```python
from build123d import *

# Parameters (mm, degrees)
F0_W     = 80
F0_H     = 25
F0_R     = 2.75
F1_DEPTH = 10
F2_R     = 4
F3_R     = 2


with BuildPart() as f1:
    # F0 (on Top) → F1 (new body)
    with BuildSketch(Plane.XY):
        Rectangle(F0_W, F0_H)
        with Locations((32.5, 0)):
            Circle(F0_R, mode=Mode.SUBTRACT)
    extrude(amount=F1_DEPTH)

    # F2
    f2_edges = [f1.edges().sort_by_distance(p)[0] for p in [
        (40, -12.5, 5),
        (-40, -12.5, 5),
        (40, 12.5, 5),
        (-40, 12.5, 5),
    ]]
    fillet(f2_edges, radius=F2_R)

    # F3
    f3_edges = [f1.edges().sort_by_distance(p)[0] for p in [
        (0, -12.5, 10),
    ]]
    fillet(f3_edges, radius=F3_R)


solid = f1.part
```
Could you check a few things on this model? Use its own coordinates, in mm. Round coordinates to 2 decimals unless told otherwise and drop trailing zeros. Loops run counter-clockwise (first coordinate to the right, second up) from the corner with the lowest first, then second, coordinate; pieces in that order, holes last.
Q1. I want a section at A-A (y = 0). Write out the boundary of the cut face in (x, z).
Q2. I want a section at C-C (z = 3.75). Write out the boundary of the cut face in (x, y), and give its area (3 significant figures).
Q3. Thinking about a two-plate mould opening in X: for faces 1 (the cylindrical face through (29.753, 0.121, 4.93)), 2 (the cylindrical face through (-39.4, -0.12, 9.43)), 3 (the cylindrical face through (-0.5, 11.9, 9.43)), which applies, pulls with the +X half, pulls with the -X half, needs draft (parallel to the pull), parting line crosses it, or undercut?
Q4. I want a section at B-B (x = 32.5). Write out the boundary of the cut face in (y, z), and give its area (3 significant figures).
Q5. For P1, Ø1.5, axis at y = -9.5, z = 5, coming from the -X side, with a flat end and sliding along its axis, tell me the tip position at first contact or that it passes through.
Q6. Please list where these lines run through material, in increasing order: L1, parallel to Y at x = 32.5, z = 8.25; L2, parallel to X at y = -0.75, z = 1.75; L3, parallel to Y at x = 30, z = 0.5.
Answer below:
1. outline: (-40, 0) - (29.75, 0) - (29.75, 10) - (-38, 10) arc R2 ccw to (-40, 8) - close; (35.25, 0) - (40, 0) - (40, 8) arc R2 ccw to (38, 10) - (35.25, 10) - close
2. outline: (-40, -8.5) arc R4 ccw to (-36, -12.5) - (36, -12.5) arc R4 ccw to (40, -8.5) - (40, 8.5) arc R4 ccw to (36, 12.5) - (-36, 12.5) arc R4 ccw to (-40, 8.5) - close; hole circle Ø5.5 at (32.5, 0)
2. area: 1,960 mm2
3. face 1: undercut
3. face 2: pulls with the -X half
3. face 3: needs draft
4. outline: (-12.5, 0) - (-2.75, 0) - (-2.75, 10) - (-10.5, 10) arc R2 ccw to (-12.5, 8) - close; (2.75, 0) - (12.5, 0) - (12.5, 8) arc R2 ccw to (10.5, 10) - (2.75, 10) - close
4. area: 193 mm2
5. P1: stops at x = -39.99
6. L1: y = -12.48 to -2.75, 2.75 to 12.48
6. L2: x = -40 to 29.85, 35.15 to 40
6. L3: y = -12.5 to -1.15, 1.15 to 12.5
